from build123d import *

# Parameters (mm, degrees)
SKETCH1_W           = 10
SKETCH1_H           = 10
BOSS_EXTRUDE1_DEPTH = 7.5


with BuildPart() as part:
    # Sketch1 → Boss-Extrude1 (new body)
    with BuildSketch(Plane.XY):
        with BuildLine():
            Line((9.931375967, 20.189144499), (24.890876528, 16.746470245))
            ThreePointArc((24.890876528, 16.746470245), (25.212386049, 16.25840059), (25.524326618, 15.764160323))
            Line((25.524326618, 15.764160323), (18.695396131, 12.518624033))
            Line((18.695396131, 12.518624033), (29.929366518, 2.057430392))
            ThreePointArc((29.929366518, 2.057430392), (29.963767103, 1.473994911), (29.986795427, 0.89))
            Line((29.986795427, 0.89), (22.45, 1.493748368))
            Line((22.45, 1.493748368), (26.94830692, -13.182896273))
            ThreePointArc((26.94830692, -13.182896273), (26.68638096, -13.705366513), (26.414326618, -14.222635104))
            Line((26.414326618, -14.222635104), (20.189144499, -9.931375967))
            Line((20.189144499, -9.931375967), (16.746470245, -24.890876528))
            ThreePointArc((16.746470245, -24.890876528), (16.25840059, -25.212386049), (15.764160323, -25.524326618))
            Line((15.764160323, -25.524326618), (12.518624033, -18.695396131))
            Line((12.518624033, -18.695396131), (2.057430392, -29.929366518))
            ThreePointArc((2.057430392, -29.929366518), (1.473994911, -29.963767103), (0.89, -29.986795427))
            Line((0.89, -29.986795427), (1.493748368, -22.45))
            Line((1.493748368, -22.45), (-13.182896273, -26.94830692))
            ThreePointArc((-13.182896273, -26.94830692), (-13.705366513, -26.68638096), (-14.222635104, -26.414326618))
            Line((-14.222635104, -26.414326618), (-9.931375967, -20.189144499))
            Line((-9.931375967, -20.189144499), (-24.890876528, -16.746470245))
            ThreePointArc((-24.890876528, -16.746470245), (-25.212386049, -16.25840059), (-25.524326618, -15.764160323))
            Line((-25.524326618, -15.764160323), (-18.695396131, -12.518624033))
            Line((-18.695396131, -12.518624033), (-29.929366518, -2.057430392))
            ThreePointArc((-29.929366518, -2.057430392), (-29.963767103, -1.473994911), (-29.986795427, -0.89))
            Line((-29.986795427, -0.89), (-22.45, -1.493748368))
            Line((-22.45, -1.493748368), (-26.94830692, 13.182896273))
            ThreePointArc((-26.94830692, 13.182896273), (-26.68638096, 13.705366513), (-26.414326618, 14.222635104))
            Line((-26.414326618, 14.222635104), (-20.189144499, 9.931375967))
            Line((-20.189144499, 9.931375967), (-16.746470245, 24.890876528))
            ThreePointArc((-16.746470245, 24.890876528), (-16.25840059, 25.212386049), (-15.764160323, 25.524326618))
            Line((-15.764160323, 25.524326618), (-12.518624033, 18.695396131))
            Line((-12.518624033, 18.695396131), (-2.057430392, 29.929366518))
            ThreePointArc((-2.057430392, 29.929366518), (-1.473994911, 29.963767103), (-0.89, 29.986795427))
            Line((-0.89, 29.986795427), (-1.493748368, 22.45))
            Line((-1.493748368, 22.45), (13.182896273, 26.94830692))
            ThreePointArc((13.182896273, 26.94830692), (13.705366513, 26.68638096), (14.222635104, 26.414326618))
            Line((14.222635104, 26.414326618), (9.931375967, 20.189144499))
        make_face()
        Rectangle(SKETCH1_W, SKETCH1_H, mode=Mode.SUBTRACT)
    extrude(amount=BOSS_EXTRUDE1_DEPTH)


solid = part.part
Read the model definition and answer for the solid it produces. Units are mm, in the model's axes. A direction names the side the tool comes from. Give positions to 0.01 mm unless a question says otherwise; leave off trailing zeros. Write each loop counter-clockwise with the first axis right and the second up, starting at its lowest first coordinate (ties: lowest second). Pieces come first, ordered by that corner, then holes. Notation, with made-up numbers: M 18.5,29.5 L 46.5,29.5 A21 cw 46.5,50.5 Z; hole C -21.5,-27 d5. An arc over 180 degrees is marked long. One line per item, written item: value. Start each with the question number.
(1) Find the intervals of material crossed by line 1 (X direction, y = -10.5, z = 1.5); line 2 (Y direction, x = 14, z = 6.25); line 3 (Y direction, x = -3.5, z = 3.5), in increasing order.
(2) Find section D-D (y = 7). Determine the outline of the cut face in (x, z).
(3) Find section C-C (x = 9). Determine the outline of the cut face in (y, z), plus the area to 3 significant figures.
(4) Find section A-A (y = -11). Determine the outline of the cut face in (x, z), plus the area to 3 significant figures.
(5) Find section B-B (x = -21.5). Determine the outline of the cut face in (y, z) (3 decimals), plus the area to 3 significant figures.
(6) Determine the mould class of faces 6 (the flat face through (-26.271, -1.188, 3.698)), 7 (the flat face through (0, -6, 0)), 8 (the flat face through (-24.234, -7.361, 3.698)) for opening direction X: pulls with the +X half, pulls with the -X half, needs draft (parallel to the pull), parting line crosses it, or undercut.
(7) A tool of negligible diameter and unlimited length cuts with its end or side. For faces 1 (the flat face through (24.234, 7.361, 3.698)), 2 (the flat face through (14.164, -22.158, 3.698)), 3 (the flat face through (-7.361, 24.234, 3.698)), 4 (the flat face through (-12.11, -23.35, 3.7)), 5 (the flat face through (-5, 0, 4)), from which of +Z, -Z, +X, -X, +Y, -Y can it reach the whole face along a straight path? Write none if from no direction.
(8) Flat-ended cylindrical pins translate along their axes: pin 1 Ø6 at (x, y) = (23, 21.5) entering from +Z; pin 2 Ø3 at (y, z) = (21.5, 5.5) entering from -X; pin 3 Ø4 at (x, z) = (14.5, 6.5) entering from +Y; pin 4 Ø1 at (y, z) = (-15.5, 1) entering from -X. Find the tip coordinate at first contact, or state that the pin passes through.
Results below:
1. line 1: x = -20.86 to 20.06, 21.01 to 26.13
1. line 2: y = -21.81 to 19.25, 26.09 to 26.53
1. line 3: y = -23.98 to -5, 5 to 28.38
2. outline: M -25.05,0 L 24.62,0 L 24.62,7.5 L -25.05,7.5 Z
3. outline: M -22.47,0 L 25.67,0 L 25.67,7.5 L -22.47,7.5 Z
3. area: 361 mm^2
4. outline: M -20.33,0 L 19.94,0 L 19.94,7.5 L -20.33,7.5 Z; M 21.74,0 L 26.28,0 L 26.28,7.5 L 21.74,7.5 Z
4. area: 336 mm^2
5. outline: M -17.527,0 L -13.852,0 L -13.852,7.5 L -17.527,7.5 Z; M -9.907,0 L 10.835,0 L 10.835,7.5 L -9.907,7.5 Z
5. area: 183 mm^2
6. face 6: undercut
6. face 7: needs draft
6. face 8: pulls with the -X half
7. face 1: +Z, -Z, +X
7. face 2: +Z, -Z, -Y
7. face 3: +Z, -Z, +Y
7. face 4: +Z, -Z, -X
7. face 5: +Z, -Z
8. pin 1: passes through
8. pin 2: stops at x = -17.87
8. pin 3: stops at y = 26.95
8. pin 4: stops at x = -25.52
